from build123d import *

# Parameters (mm, degrees)
ESQUISSE1_W        = 40
ESQUISSE1_H        = 100
BOSS_EXTRU_1_DEPTH = 40
BOSS_EXTRU_2_DEPTH = 20


with BuildPart() as part:
    # Esquisse1 → Boss.-Extru.1 (new body)
    with BuildSketch(Plane(origin=(0, 0, 0), x_dir=(1, 0, 0), z_dir=(0, 1, 0))):
        with Locations((20, 50)):
            Rectangle(ESQUISSE1_W, ESQUISSE1_H)
    extrude(amount=BOSS_EXTRU_1_DEPTH)

    # Esquisse2 → Boss.-Extru.2 (add)
    with BuildSketch(Plane.XY):
        Polygon((23, 28.267949192), (23, 31.732050808), (20, 33.464101615), (17, 31.732050808), (17, 28.267949192), (20, 26.535898385), align=None)
    extrude(amount=BOSS_EXTRU_2_DEPTH)


solid = part.part
Verification items for the finished model (mm, model axes). A direction names the side the tool comes from. Coordinates: 2 decimals unless noted, no trailing zeros. Order: outer loops, then holes, each group sorted by start corner. A loop starts at its lowest first (then second) coordinate and runs counter-clockwise, first axis right, second up. Notation, with made-up numbers: M 68.25,9.5 L 116.25,9.5 A9 ccw 116.25,26.5 Z; hole C -18,44.25 d11. An arc over 180 degrees is marked long. One line per item, written item: value. Start each with the question number.
Item 1: Access from +Z, -Z, +X, -X, +Y, -Y to the whole of each face (thin tool, end or side, straight path). Record for faces 1 (the flat face through (18.5, 27.4, 9.9)), 2 (the flat face through (21.5, 32.6, 9.9)), 3 (the flat face through (21.5, 27.4, 9.9)).
Item 2: Depth check by flat-ended pin: P1, Ø3, axis at y = 30, z = 5, coming from the +X side; P2, Ø4, axis at x = 30, y = 17.5, coming from the +Z side; P3, Ø3, axis at y = 30, z = 11.5, coming from the -X side. Enter the tip coordinate at first touch or a pass-through.
Item 3: Sectioned sample at B-B on y = 13.5. Record the cut outline in (x, z).
Item 4: Sectioned sample at A-A on z = 7.5. Record the cut outline in (x, y).
Item 5: Thickness scan on probe 1 along Z at (x, y) = (31, 22); probe 2 along Y at (x, z) = (17.5, 10.5). Record the ranges inside material, lowest first.
Calculated:
1. face 1: +Z, -X, -Y
1. face 2: +Z, +X, +Y
1. face 3: +Z, +X, -Y
2. P1: x = 23
2. P2: z = 0
2. P3: x = 17
3. outline: M 0,-100 L 40,-100 L 40,0 L 0,0 Z
4. outline: M 17,28.27 L 20,26.54 L 23,28.27 L 23,31.73 L 20,33.46 L 17,31.73 Z
5. probe 1: -100 to 0
5. probe 2: 27.98 to 32.02
